Part print with two shaded views. Sizes in mm from the minimum x, y, z corner. A direction names the side the tool comes from. Round coordinates to 2 decimals unless told otherwise and drop trailing zeros. Loops run counter-clockwise (first coordinate to the right, second up) from the corner with the lowest first, then second, coordinate; pieces in that order, holes last. Notation, with made-up numbers: M -27.5,77.25 L 23.5,77.25 A37 cw 23.5,114.25 Z; hole C 68,12 d1. An arc over 180 degrees is marked long. Answer as CSV lines item,"result". Start each with the question number.
Item 1: Band-saw the part on D-D (z = 5.75). Give the cut face in (x, y), and give its area (3 significant figures).
Item 2: Wall check: line 1 (X direction, y = 3.5, z = 3); line 2 (X direction, y = 7.25, z = 4); line 3 (Z direction, x = 5, y = 2.5). Give the ranges that are in metal, low to high.
Item 3: Drop flat-ended pins along their axis: pin 1 Ø2.5 at (x, z) = (32, 4.5) entering from +Y; pin 2 Ø1.5 at (x, z) = (24, 6.5) entering from +Y; pin 3 Ø0.9 at (y, z) = (8.5, 3) entering from +X. Give the stop position or say it passes through.
Item 4: Band-saw the part on B-B (y = 7.5). Give the cut face in (x, z), and give its area (3 significant figures).
Item 5: Band-saw the part on C-C (x = 5). Give the cut face in (y, z), and give its area (3 significant figures).
Item 6: Mould opens along X. For the marked faces 1, 2 and 3 say: pulls with the +X half, pulls with the -X half, needs draft (parallel to the pull), parting line crosses it, or undercut.
Item 7: Which spindle directions (+Z, -Z, +X, -X, +Y, -Y) get a long thin tool onto all of the face, cutting with end or side? Do the marked faces 4, 5, 6 and 7. Say none if no direction does.
Item 8: Band-saw the part on A-A (y = 4.5). Give the cut face in (x, z), and give its area (3 significant figures).
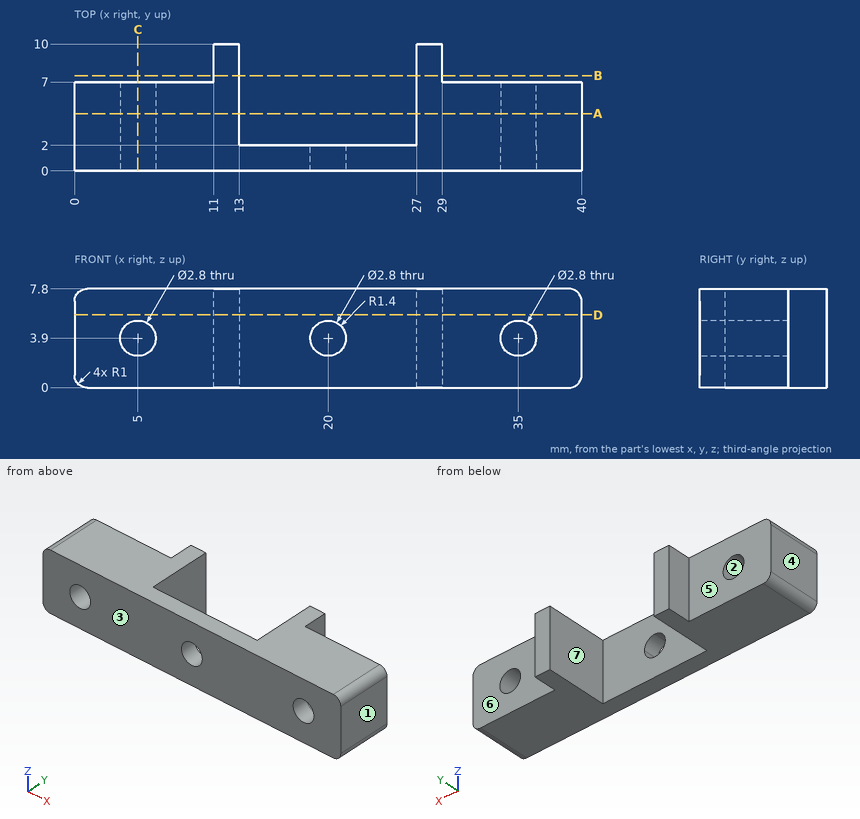
Answer block:
1,outline,"M 0,0 L 40,0 L 40,7 L 29,7 L 29,10 L 27,10 L 27,2 L 13,2 L 13,10 L 11,10 L 11,7 L 0,7 Z"
1,area,"222 mm^2"
2,line 1,"x = 0 to 3.93, 6.07 to 13, 27 to 33.93, 36.07 to 40"
2,line 2,"x = 11 to 13, 27 to 29"
2,line 3,"z = 0 to 2.5, 5.3 to 7.8"
3,pin 1,"stops at y = 7"
3,pin 2,"stops at y = 2"
3,pin 3,"stops at x = 29"
4,outline,"M 11,0 L 13,0 L 13,7.8 L 11,7.8 Z; M 27,0 L 29,0 L 29,7.8 L 27,7.8 Z"
4,area,"31.2 mm^2"
5,outline,"M 0,0 L 7,0 L 7,2.5 L 0,2.5 Z; M 0,5.3 L 7,5.3 L 7,7.8 L 0,7.8 Z"
5,area,"35.0 mm^2"
6,face 1,"pulls with the +X half"
6,face 2,"undercut"
6,face 3,"needs draft"
7,face 4,"+Z, -Z, -X, +Y, -Y"
7,face 5,"+Z, -Z, -X, +Y"
7,face 6,"+Z, -Z, +X, +Y"
7,face 7,"+Z, -Z, +Y"
8,outline,"M 0,1 A1 ccw 1,0 L 13,0 L 13,7.8 L 1,7.8 A1 ccw 0,6.8 Z; M 27,0 L 39,0 A1 ccw 40,1 L 40,6.8 A1 ccw 39,7.8 L 27,7.8 Z; hole C 5,3.9 d2.8; hole C 35,3.9 d2.8"
8,area,"190 mm^2"
